Solid Edge part; units mm, degrees
sketch "Sketch1" plane through (0, 0, 0) normal (0, 0, 1) x (1, 0, 0)
  line L0 (0, -4.0415) -> (3.5, -2.0207)
  line L1 (3.5, -2.0207) -> (3.5, 2.0207)
  line L2 (3.5, 2.0207) -> (0, 4.0415)
  line L3 (0, 4.0415) -> (-3.5, 2.0207)
  line L4 (-3.5, 2.0207) -> (-3.5, -2.0207)
  line L5 (-3.5, -2.0207) -> (0, -4.0415)
extrude "Protrusion1" add sketch "Sketch1" along normal blind 2.5
sketch "Sketch2" plane through (0, 0, 0) normal (0, 0, -1) x (0.866, 0.5, 0)
  circle A0 centre (0, 0) radius 5
extrude "ExtrudedProtrusion_2" add sketch "Sketch2" along normal blind 0.5
extrude "Protrusion2" [suppressed]
sketch "Sketch3" plane through (0, 0, 0) normal (0, -1, 0) x (1, 0, 0)
  line L0 (7.8301, 2.5) -> (3.5, 2.5)
  line L1 (3.5, 2.5) -> (7.8301, 0)
  line L2 (7.8301, 0) -> (7.8301, 2.5)
revolve "RevolvedCutout1" cut sketch "Sketch3" angle 360 about axis through (0, 0, 10.8167) along (0, 0, -1)
sketch "Sketch4" plane through (0, 0, 0) normal (0, 0, 1) x (1, 0, 0)
  circle A0 centre (0, 0.0203) radius 2.5
extrude "Protrusion3" add sketch "Sketch4" against normal blind 10
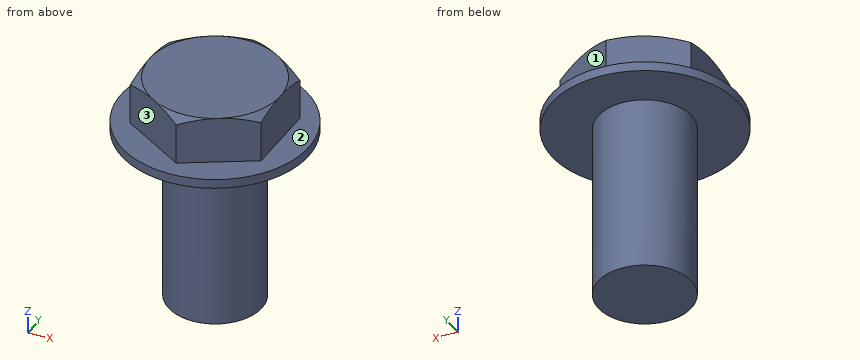
Input: part model. Units: mm. Frame: model coordinates. Face numbers are marked on the shaded views. A direction names the side the tool comes from. Give positions to 0.01 mm unless a question says otherwise; leave off trailing zeros. Order: outer loops, then holes, each group sorted by start corner. A loop starts at its lowest first (then second) coordinate and runs counter-clockwise, first axis right, second up. Notation, with made-up numbers: (-34.75, 89) - (14.25, 89) arc R12 cw to (14.25, 95) - close; hole circle Ø5 at (85.5, 22.5). An arc over 180 degrees is marked (long way). Put each result on its own line as item: value.
Item 1: Section query C-C, the plane z = -2.25. Return loops of the section in (x, y), then the cut area to 3 significant figures.
Found:
outline: circle Ø5 at (0, 0.02)
area: 19.6 mm^2
Item 2: Ray query, L1, parallel to Z at x = 1, y = 4; L2, parallel to Y at x = 0, z = -8.75; L3, parallel to Z at x = 2.75, y = 1.5. Return the intervals inside material, ascending. Write a range as from..to.
Found:
L1: z = -0.5..0
L2: y = -2.48..2.52
L3: z = -0.5..2.5
Item 3: Section query A-A, the plane z = 0.25. Return loops of the section in (x, y), then the cut area to 3 significant figures.
Found:
outline: (-3.5, -2.02) - (0, -4.04) - (3.5, -2.02) - (3.5, 2.02) - (0, 4.04) - (-3.5, 2.02) - close
area: 42.4 mm^2
Item 4: Contact query for flat-ended pins moving along their axis: pin 1 (3 mm diameter, centred on y = 1.5, z = -4.5, fed in from -X); pin 2 (3 mm diameter, centred on x = 1.5, z = -4.5, fed in from -Y); pin 3 (1.2 mm diameter, centred on y = 0, z = 1.5, fed in from +X). Output: stop coordinate, or through.
Found:
pin 1: stops at x = -2.5
pin 2: stops at y = -2.48
pin 3: stops at x = 3.5
Item 5: Section query B-B, the plane y = -4.25. Return loops of the section in (x, z), then the cut area to 3 significant figures.
Found:
outline: (-2.63, -0.5) - (2.63, -0.5) - (2.63, 0) - (-2.63, 0) - close
area: 2.63 mm^2
Item 6: Access query for the marked faces 1, 2 and 3. Directions: +Z, -Z, +X, -X, +Y, -Y. A direction counts if a zero-diameter tool reaches every point of the face in a straight line with its end or side. Return the directions, or none.
Found:
face 1: +Z, +X, +Y
face 2: +Z
face 3: +Z, -X, -Y
